Can you work these out from the model? Positions are in its coordinate system, mm. Face numbers are marked on the shaded views. A direction names the side the tool comes from. Coordinates: 2 decimals unless noted, no trailing zeros. Order: outer loops, then holes, each group sorted by start corner. A loop starts at its lowest first (then second) coordinate and runs counter-clockwise, first axis right, second up. Notation, with made-up numbers: (-11, 28.5) -> (27, 28.5) arc R25 ccw to (27, 44.5) -> close; hole circle Ø7 at (-12.75, 71). An arc over 180 degrees is marked (long way). Use a Markdown table: item, result. Add a question column.
1. For pin 1 Ø2.5 at (x, y) = (0, 7.5) entering from -Z; pin 2 Ø1 at (x, y) = (6.5, 6) entering from +Z; pin 3 Ø0.9 at (x, y) = (7.5, 0) entering from -Z; pin 4 Ø1 at (x, z) = (-4, -4.5) entering from -Y, each with a flat end and sliding along its axis, tell me the tip position at first contact or that it passes through.
2. Suppose I cut it at C-C, the plane z = -2.5. List the corners of the cut face in (x, y) for me.
3. We'd pull the mould along X, two halves only. Please class the marked faces 1, 2 and 3: pulls with the +X half, pulls with the -X half, needs draft (parallel to the pull), parting line crosses it, or undercut.
4. For the marked faces 4 and 5, which set-ups out of +Z, -Z, +X, -X, +Y, -Y let a thin tool reach every point of the face, with its end or its side?
5. Suppose I cut it at A-A, the plane y = 0. State how many separate pieces and enclosed holes the cut face has, then the cut area to 3 significant figures.
6. Suppose I cut it at D-D, the plane x = -7.5. List the corners of the cut face in (y, z) for me.
7. If I drill on line 1 along Y through (x, z) = (0, -0.4); line 2 along Y through (x, z) = (-7.5, -1.3); line 3 along Y through (x, z) = (-3.8, -0.45), over which ranges is the centre line in solid material (lowest first)? Write a range as from..to.
```python
from build123d import *

# Parameters (mm, degrees)
F0_R     = 10.5
F0_R_2   = 0.75
F0_R_3   = 3.5
F0_R_4   = 3
F1_DEPTH = 2
F2_DEPTH = 1
F3_R     = 4
F4_DEPTH = 4
F6_D     = 4.4
F8_D     = 6
F8_DEPTH = 4
F8_TIP   = 1.8025818571


with BuildPart() as f1:
    # F0 (on Top) → F1 (new body)
    with BuildSketch(Plane.XY):
        Circle(F0_R)
        with Locations((-3.8, -7.5)):
            Circle(F0_R_2, mode=Mode.SUBTRACT)
        with Locations((-7.5, -3.8)):
            Circle(F0_R_2, mode=Mode.SUBTRACT)
        with Locations((0, -7.5)):
            Circle(F0_R_2, mode=Mode.SUBTRACT)
        with Locations((3.8, -7.5)):
            Circle(F0_R_2, mode=Mode.SUBTRACT)
        with Locations((7.5, -3.8)):
            Circle(F0_R_2, mode=Mode.SUBTRACT)
        with Locations((-7.5, 0)):
            Circle(F0_R_2, mode=Mode.SUBTRACT)
        with Locations((-7.5, 3.8)):
            Circle(F0_R_2, mode=Mode.SUBTRACT)
        with Locations((-3.8, 7.5)):
            Circle(F0_R_2, mode=Mode.SUBTRACT)
        Circle(F0_R_3, mode=Mode.SUBTRACT)
        with Locations((7.5, 0)):
            Circle(F0_R_2, mode=Mode.SUBTRACT)
        with Locations((7.5, 3.8)):
            Circle(F0_R_2, mode=Mode.SUBTRACT)
        with Locations((0, 7.5)):
            Circle(F0_R_2, mode=Mode.SUBTRACT)
        with Locations((3.8, 7.5)):
            Circle(F0_R_2, mode=Mode.SUBTRACT)
        Circle(F0_R_3)
        Circle(F0_R_4, mode=Mode.SUBTRACT)
        Circle(F0_R_4)
    extrude(amount=-F1_DEPTH)

    # F0 (on Top) → F2 (join)
    with BuildSketch(Plane.XY):
        Circle(F0_R_3)
        Circle(F0_R_4, mode=Mode.SUBTRACT)
    extrude(amount=F2_DEPTH)

    # F3 (on face) → F4 (join)
    with BuildSketch(Plane(origin=(0, 0, -2), x_dir=(1, 0, 0), z_dir=(0, 0, -1))):
        Circle(F3_R)
    extrude(amount=F4_DEPTH)

    # F6 (through all)
    with Locations(Plane.XY):
        with Locations((0, 0)):
            Hole(F6_D / 2)

    # F8
    with Locations(Plane(origin=(0, 0, -6), x_dir=(1, 0, 0), z_dir=(0, 0, -1))):
        with Locations((0, 0)):
            Hole(F8_D / 2, depth=F8_DEPTH)
            with Locations((0, 0, -(F8_DEPTH + F8_TIP / 2))):  # 118° drill point
                Cone(0, F8_D / 2, F8_TIP, mode=Mode.SUBTRACT)


solid = f1.part
```
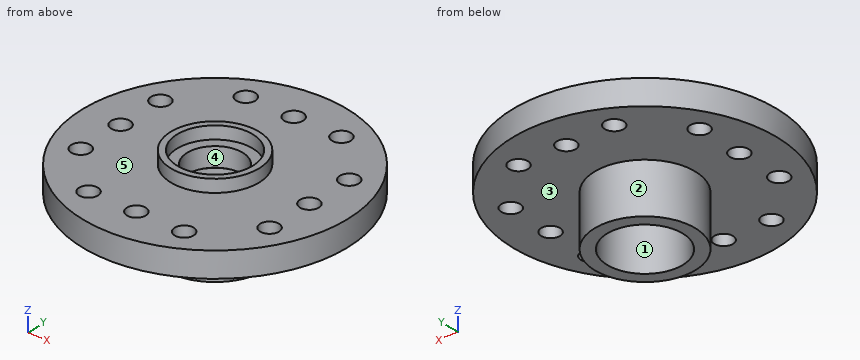
Worked out:
| question | item | result |
|---|---|---|
| 1 | pin 1 | stops at z = -2 |
| 1 | pin 2 | stops at z = 0 |
| 1 | pin 3 | passes through |
| 1 | pin 4 | stops at y = -1.94 |
| 2 | outline | circle Ø8 at (0, 0); hole circle Ø6 at (0, 0) |
| 3 | face 1 | undercut |
| 3 | face 2 | parting line crosses it |
| 3 | face 3 | needs draft |
| 4 | face 4 | +Z, -Z |
| 4 | face 5 | +Z |
| 5 | separate pieces | 4 |
| 5 | enclosed holes | 0 |
| 5 | area | 35.8 mm² |
| 6 | outline | (-7.35, -2) -> (-4.55, -2) -> (-4.55, 0) -> (-7.35, 0) -> close; (-3.05, -2) -> (-0.75, -2) -> (-0.75, 0) -> (-3.05, 0) -> close; (0.75, -2) -> (3.05, -2) -> (3.05, 0) -> (0.75, 0) -> close; (4.55, -2) -> (7.35, -2) -> (7.35, 0) -> (4.55, 0) -> close |
| 7 | line 1 | y = -10.5..-8.25, -6.75..-2.2, 2.2..6.75, 8.25..10.5 |
| 7 | line 2 | y = -7.35..-4.55, -3.05..-0.75, 0.75..3.05, 4.55..7.35 |
| 7 | line 3 | y = -9.79..-8.25, -6.75..6.75, 8.25..9.79 |
